Here's the drawing with two shaded views (mm, measured from the low corner). I have some questions. A direction names the side the tool comes from. Give positions to 0.01 mm unless a question says otherwise; leave off trailing zeros. Loops run counter-clockwise (first coordinate to the right, second up) from the corner with the lowest first, then second, coordinate; pieces in that order, holes last. Notation, with made-up numbers: (-21.75, -7.5) - (5.25, -7.5) arc R20 ccw to (5.25, 16.5) - close; hole circle Ø11 at (-33, 18). An arc over 180 degrees is marked (long way). Answer as a JSON object with one key per item and string values. Group by question number.
Item 1: Which directions (+Z, -Z, +X, -X, +Y, -Y) give clear straight access to the entire face, cutting with the end or side of a thin tool? Please do the marked faces 1, 2, 3, 4 and 5.
Item 2: Please list where these lines run through material, in increasing order: L1, parallel to Z at x = 30, y = 11; L2, parallel to Y at x = 12, z = 8; L3, parallel to Z at x = 12.5, y = 10.5.
Item 3: Suppose I cut it at D-D on z = 3. Write out the boundary of the cut face in (x, y).
Item 4: Suppose I cut it at B-B on x = 16.5. Write out the boundary of the cut face in (y, z).
Item 5: Suppose I cut it at C-C on y = 12.75. Write out the boundary of the cut face in (x, z), and give its area (3 significant figures).
Item 6: Will these pins go through, and if not, where does the flat tip stop? pin 1 (4 mm diameter, centred on x = 27.5, y = 15.5, fed in from -Z); pin 2 (3 mm diameter, centred on y = 13, z = 5, fed in from +X); pin 3 (2.5 mm diameter, centred on y = 2, z = 13.5, fed in from -X); pin 4 (5 mm diameter, centred on x = 15, z = 6, fed in from -Y).
Item 7: Suppose I cut it at A-A on z = 12.5. Write out the boundary of the cut face in (x, y), and give its area (3 significant figures).
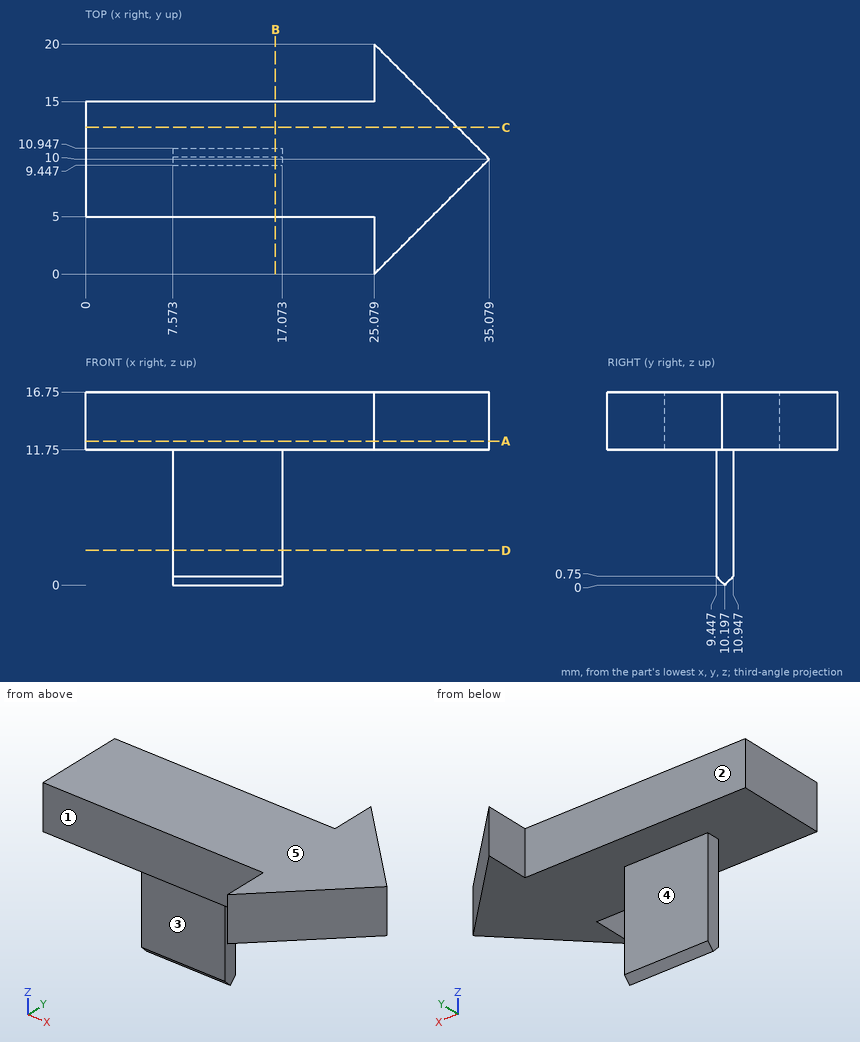
Worked out:
{
 "1": {"face 1": "+Z, -Z, -X, -Y", "face 2": "+Z, -Z, -X, +Y", "face 3": "-Z, +X, -X, -Y", "face 4": "-Z, +X, -X, +Y", "face 5": "+Z, +X, -X, +Y, -Y"},
 "2": {"L1": "z = 11.75 to 16.75", "L2": "y = 9.45 to 10.95", "L3": "z = 0.3 to 16.75"},
 "3": {"outline": "(7.57, 9.45) - (17.07, 9.45) - (17.07, 10.95) - (7.57, 10.95) - close"},
 "4": {"outline": "(5, 11.75) - (9.45, 11.75) - (9.45, 0.75) - (10.2, 0) - (10.95, 0.75) - (10.95, 11.75) - (15, 11.75) - (15, 16.75) - (5, 16.75) - close"},
 "5": {"outline": "(0, 11.75) - (32.33, 11.75) - (32.33, 16.75) - (0, 16.75) - close", "area": "162 mm2"},
 "6": {"pin 1": "stops at z = 11.75", "pin 2": "passes through", "pin 3": "stops at x = 25.08", "pin 4": "stops at y = 9.45"},
 "7": {"outline": "(0, 5) - (25.08, 5) - (25.08, 0) - (35.08, 10) - (25.08, 20) - (25.08, 15) - (0, 15) - close", "area": "351 mm2"}
}
